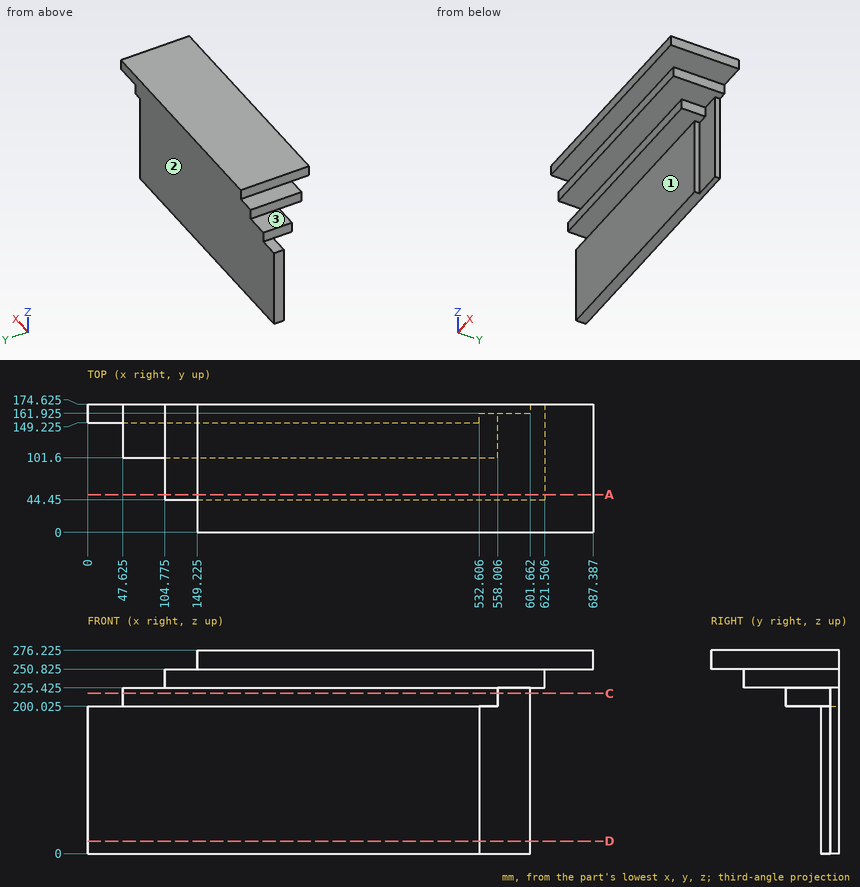
Design review of the part shown in the three views and the two pictorial views. Dimensions are in mm from the part's minimum x, y and z. A direction names the side the tool comes from. Round coordinates to 2 decimals unless told otherwise and drop trailing zeros. Loops run counter-clockwise (first coordinate to the right, second up) from the corner with the lowest first, then second, coordinate; pieces in that order, holes last. Notation, with made-up numbers: M 34,-23.5 L 86,-23.5 A24 cw 86,13.5 Z; hole C -38.75,79 d1. An arc over 180 degrees is marked long. Answer as a JSON object with one key per item and string values.
Item 1: Clearance check with flat-ended pins moving along their axes: P1, Ø10, axis at x = 557.5, z = 208, coming from the -Y side; P2, Ø13.5, axis at x = 117, y = 103, coming from the +Z side (1 decimal); P3, Ø5, axis at y = 153, z = 242.5, coming from the +X side; P4, Ø20.5, axis at y = 87.5, z = 243.5, coming from the +X side. State where each tip first meets the part, or that it passes through.
Answer sheet:
{"P1": "stops at y = 101.6", "P2": "stops at z = 250.8", "P3": "stops at x = 621.51", "P4": "stops at x = 687.39"}
Item 2: We need section A-A on y = 51.5. Give the boundary of the cut face in (x, z) (1 decimal), and give its area (3 significant figures).
Answer sheet:
{"outline": "M 104.8,225.4 L 621.5,225.4 L 621.5,250.8 L 687.4,250.8 L 687.4,276.2 L 149.2,276.2 L 149.2,250.8 L 104.8,250.8 Z", "area": "26,800 mm^2"}
Item 3: We need section C-C on z = 218. Give the boundary of the cut face in (x, y) (1 decimal), and give its area (3 significant figures).
Answer sheet:
{"outline": "M 47.6,101.6 L 558,101.6 L 558,161.9 L 601.7,161.9 L 601.7,174.6 L 47.6,174.6 Z", "area": "37,800 mm^2"}
Item 4: Wall thickness on L1, parallel to Z at x = 217.5, y = 105.5 (1 decimal); L2, parallel to Y at x = 122.5, z = 133 (1 decimal); L3, parallel to Z at x = 387.5, y = 12 (1 decimal): over which ranges is each line inside the solid? List them lowest first. Write a range as from..to.
Answer sheet:
{"L1": "z = 200..276.2", "L2": "y = 149.2..174.6", "L3": "z = 250.8..276.2"}
Item 5: Machinability: for the marked faces 1, 2 and 3, which of the approach directions +Z, -Z, +X, -X, +Y, -Y give a long, thin tool a straight path to every point of the face, cutting with its end or side? Answer none if there is none.
Answer sheet:
{"face 1": "-Z, +X, -X, -Y", "face 2": "+Z, -Z, +X, -X, +Y", "face 3": "+Z, -X, +Y, -Y"}
Item 6: We need section D-D on z = 17. Give the boundary of the cut face in (x, y) (1 decimal).
Answer sheet:
{"outline": "M 0,149.2 L 532.6,149.2 L 532.6,161.9 L 601.7,161.9 L 601.7,174.6 L 0,174.6 Z"}
